Input: part model. Units: mm. Frame: model coordinates. Round coordinates to 2 decimals unless told otherwise and drop trailing zeros. Loops run counter-clockwise (first coordinate to the right, second up) from the corner with the lowest first, then second, coordinate; pieces in that order, holes last.
(1) Cut plane C-C, the plane x = 205. Output: boundary loops of the cut face in (y, z), and give its area (3 significant figures).
(2) Cut plane D-D, the plane y = -0.6. Give the number of separate pieces and of enclosed holes in the cut face, and give its area (3 significant figures).
(3) Line query: line 1 (Z direction, x = 173, y = -1.35); line 2 (Z direction, x = 161, y = -0.7); line 3 (Z direction, x = 183.5, y = -2.7). Output: solid intervals per line, ascending.
(4) Draft query along Z for faces 1 (the face through (177.171, -1.479, 263.552)), 2 (the face through (235.278, -1.479, 183.004)), 3 (the face through (188, 0, 174)). Return one class per face: released by +Z, released by -Z, zero draft, split by the parting line, or undercut.
(5) Cut plane A-A, the plane x = 139.5. Output: boundary loops of the cut face in (y, z), and give its area (3 significant figures).
(6) Cut plane B-B, the plane z = 114. Output: boundary loops of the cut face in (x, y), and give its area (3 significant figures).
from build123d import *

# Parameters (mm, degrees)
F0_R     = 84
F0_R_2   = 20.25
F1_DEPTH = 3


# Not quite as in the source:
# - a feature of the source that left no trace in its solid (it failed there, or was rolled back) is left out


with BuildPart() as f1:
    # F0 (on Front) → F1 (new body)
    with BuildSketch(Plane.XZ):
        with Locations((188.1058226409, 180.2671665321)):
            Circle(F0_R)
        with Locations((147.5744029219, 131.9637014691)):
            Circle(F0_R_2, mode=Mode.SUBTRACT)
        with Locations((126.008084946, 169.3176599356)):
            Circle(F0_R_2, mode=Mode.SUBTRACT)
        with Locations((188.1058226409, 117.2114711388)):
            Circle(F0_R_2, mode=Mode.SUBTRACT)
        with Locations((228.6372423598, 131.9637014691)):
            Circle(F0_R_2, mode=Mode.SUBTRACT)
        with Locations((167.5180891549, 167.7861717837)):
            Circle(F0_R_2, mode=Mode.SUBTRACT)
        with Locations((209.2085479005, 168.6781637011)):
            Circle(F0_R_2, mode=Mode.SUBTRACT)
        with Locations((250.2035603357, 169.3176599356)):
            Circle(F0_R_2, mode=Mode.SUBTRACT)
        with Locations((133.497988577, 211.7950142288)):
            Circle(F0_R_2, mode=Mode.SUBTRACT)
        with Locations((187.5908308672, 204.3371641115)):
            Circle(F0_R_2, mode=Mode.SUBTRACT)
        with Locations((242.7136567047, 211.7950142288)):
            Circle(F0_R_2, mode=Mode.SUBTRACT)
        with Locations((166.539504665, 239.5201381917)):
            Circle(F0_R_2, mode=Mode.SUBTRACT)
        with Locations((209.6721406168, 239.5201381917)):
            Circle(F0_R_2, mode=Mode.SUBTRACT)
    extrude(amount=F1_DEPTH)


solid = f1.part
Reported:
1. outline: (-3, 97.98) - (0, 97.98) - (0, 106.05) - (-3, 106.05) - close; (-3, 128.38) - (0, 128.38) - (0, 148.87) - (-3, 148.87) - close; (-3, 188.49) - (0, 188.49) - (0, 193.99) - (-3, 193.99) - close; (-3, 214.68) - (0, 214.68) - (0, 219.82) - (-3, 219.82) - close; (-3, 259.22) - (0, 259.22) - (0, 262.55) - (-3, 262.55) - close
1. area: 128 mm2
2. separate pieces: 1
2. enclosed holes: 12
2. area: 6,710 mm2
3. line 1: z = 97.64 to 103.73, 130.7 to 148.29, 187.28 to 190.3, 218.38 to 220.33, 258.71 to 262.9
3. line 2: z = 100.76 to 116.8, 147.12 to 148.61, 186.96 to 220.04, 259 to 259.77
3. line 3: z = 96.39 to 97.49, 136.93 to 155.35, 180.22 to 184.5, 224.17 to 228.46, 250.58 to 264.14
4. face 1: split by the parting line
4. face 2: undercut
4. face 3: zero draft
5. outline: (-3, 111.76) - (0, 111.76) - (0, 113.39) - (-3, 113.39) - close; (-3, 150.53) - (0, 150.53) - (0, 154.22) - (-3, 154.22) - close; (-3, 184.42) - (0, 184.42) - (0, 192.45) - (-3, 192.45) - close; (-3, 231.14) - (0, 231.14) - (0, 248.78) - (-3, 248.78) - close
5. area: 93.0 mm2
6. outline: (136.49, -3) - (138.23, -3) - (138.23, 0) - (136.49, 0) - close; (156.92, -3) - (168.11, -3) - (168.11, 0) - (156.92, 0) - close; (208.1, -3) - (219.29, -3) - (219.29, 0) - (208.1, 0) - close; (237.98, -3) - (239.73, -3) - (239.73, 0) - (237.98, 0) - close
6. area: 77.6 mm2
